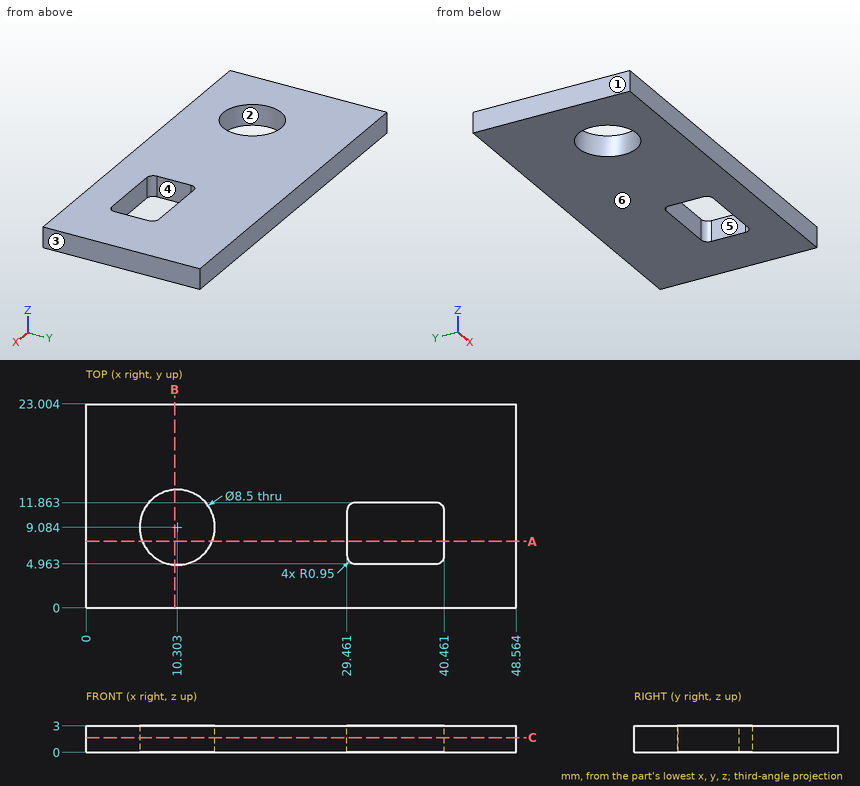
Job drawing, mm, ordinate dimensions from the low corner. One solid piece. A direction names the side the tool comes from. Round coordinates to 2 decimals unless told otherwise and drop trailing zeros. Write each loop counter-clockwise with the first axis right and the second up, starting at its lowest first coordinate (ties: lowest second). Pieces come first, ordered by that corner, then holes.
1) Band-saw the part on A-A, the plane y = 7.5. List the corners of the cut face in (x, z).
2) 3-axis set-ups, long thin cutter, end or side, ignore diameter. For the marked faces 5 and 6: which of +Z, -Z, +X, -X, +Y, -Y reach the whole face in a straight line?
3) Mould opens along X. For the marked faces 1, 2, 3 and 4 say: +X half, -X half, draft (parallel to the pull), parting line (faces both ways), or undercut.
4) Band-saw the part on C-C, the plane z = 1.65. List the corners of the cut face in (x, y), and give its area (3 significant figures).
5) Band-saw the part on B-B, the plane x = 10. List the corners of the cut face in (y, z) (1 decimal).
6) Drill centre lines: probe 1 along Y at (x, z) = (35.5, 2.6); probe 2 along X at (y, z) = (8.25, 2.4) (1 decimal); probe 3 along X at (y, z) = (6.5, 2.5) (1 decimal). Where is each one in solid material? Low to high.
Ans:
1. outline: (0, 0) - (6.36, 0) - (6.36, 3) - (0, 3) - close; (14.25, 0) - (29.46, 0) - (29.46, 3) - (14.25, 3) - close; (40.46, 0) - (48.56, 0) - (48.56, 3) - (40.46, 3) - close
2. face 5: +Z, -Z
2. face 6: -Z, +X, -X, +Y, -Y
3. face 1: -X half
3. face 2: undercut
3. face 3: +X half
3. face 4: undercut
4. outline: (0, 0) - (48.56, 0) - (48.56, 23) - (0, 23) - close; hole circle Ø8.5 at (10.3, 9.08); hole (29.46, 5.91) arc R0.95 ccw to (30.41, 4.96) - (39.51, 4.96) arc R0.95 ccw to (40.46, 5.91) - (40.46, 10.91) arc R0.95 ccw to (39.51, 11.86) - (30.41, 11.86) arc R0.95 ccw to (29.46, 10.91) - close
4. area: 985 mm2
5. outline: (0, 0) - (4.8, 0) - (4.8, 3) - (0, 3) - close; (13.3, 0) - (23, 0) - (23, 3) - (13.3, 3) - close
6. probe 1: y = 0 to 4.96, 11.86 to 23
6. probe 2: x = 0 to 6.1, 14.5 to 29.5, 40.5 to 48.6
6. probe 3: x = 0 to 6.9, 13.7 to 29.5, 40.5 to 48.6
